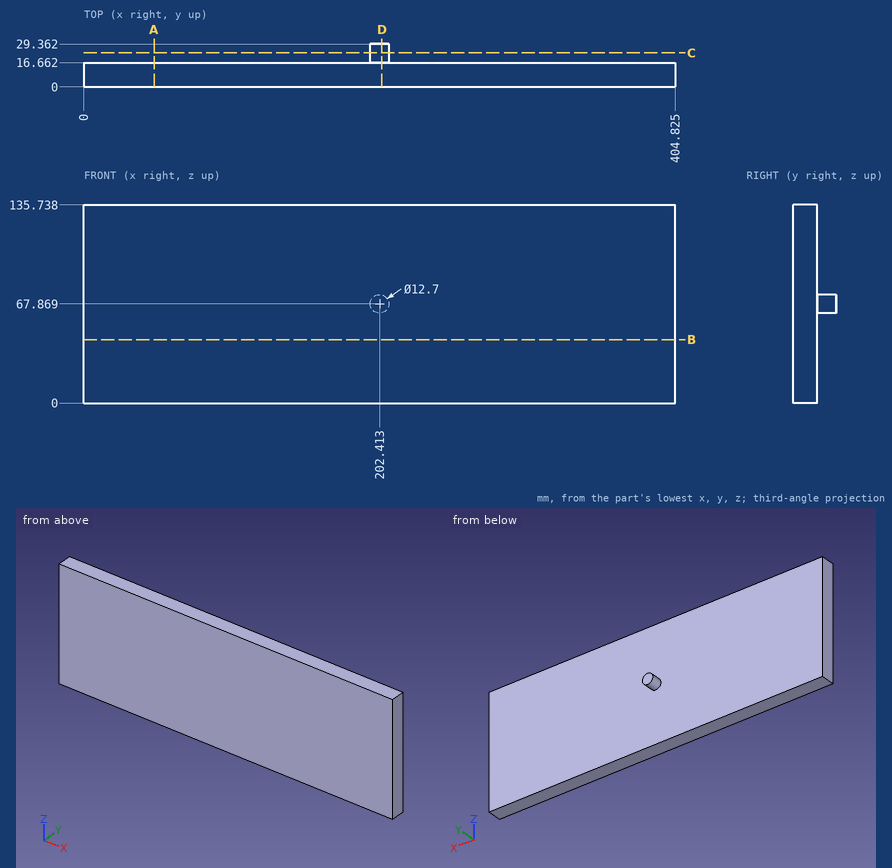
Answer from the drawing. Dimensions are ordinates in mm from the lowest x, y and z of the part. Give positions to 0.01 mm unless a question says otherwise; leave off trailing zeros. Write each loop counter-clockwise with the first axis right and the second up, starting at its lowest first coordinate (ties: lowest second). Pieces come first, ordered by that corner, then holes. Notation, with made-up numbers: (70, 9.25) - (119, 9.25) arc R11 ccw to (119, 20.25) - close; hole circle Ø7 at (-24.5, 85.25). An arc over 180 degrees is marked (long way). One line per item, written item: value. Start each with the question number.
1. Consider probe 1 along Y at (x, z) = (348.5, 75); probe 2 along X at (y, z) = (16.75, 64). Determine where each line is inside the solid, lowest interval first.
2. Find section C-C (y = 23.25). Write down the section's boundary in (x, z), then the cut area to 3 significant figures.
3. Find section A-A (x = 48). Write down the section's boundary in (y, z).
4. Find section D-D (x = 204). Write down the section's boundary in (y, z), then the cut area to 3 significant figures.
5. Find section B-B (z = 43.5). Write down the section's boundary in (x, y) (1 decimal).
6. Given pin 1 (1.5 mm diameter, centred on x = 179.5, z = 121, fed in from +Y), flat-ended and moving along its own axis, determine where the tip first touches the part or whether it passes through.
Geometry results:
1. probe 1: 0 to 16.66
1. probe 2: 197.38 to 207.45
2. outline: circle Ø12.7 at (202.41, 67.87)
2. area: 127 mm2
3. outline: (0, 0) - (16.66, 0) - (16.66, 135.74) - (0, 135.74) - close
4. outline: (0, 0) - (16.66, 0) - (16.66, 61.72) - (29.36, 61.72) - (29.36, 74.02) - (16.66, 74.02) - (16.66, 135.74) - (0, 135.74) - close
4. area: 2,420 mm2
5. outline: (0, 0) - (404.8, 0) - (404.8, 16.7) - (0, 16.7) - close
6. pin 1: y = 16.66
